```python
from build123d import *

# Parameters (mm, degrees)
BOSS_EXTRUDE1_DEPTH = 1.5
SKETCH3_W           = 30
SKETCH3_H           = 3
BOSS_EXTRUDE2_DEPTH = 3
SKETCH5_W           = 20
SKETCH5_H           = 3
BOSS_EXTRUDE3_DEPTH = 3


with BuildPart() as part:
    # Sketch2 → Boss-Extrude1 (new, symmetric)
    with BuildSketch(Plane.XY):
        with BuildLine():
            Line((-209.776110705, -9.374567854), (-209.776110705, 10.625432146))
            ThreePointArc((-209.776110705, 10.625432146), (-193.252620605, 27.63865465), (-170.374325813, 33.888382039))
            Line((-170.374325813, 33.888382039), (200.822104404, 33.888382039))
            ThreePointArc((200.822104404, 33.888382039), (223.700399196, 27.63865465), (240.223889295, 10.625432146))
            Line((240.223889295, 10.625432146), (240.223889295, -9.374567854))
            Line((240.223889295, -9.374567854), (-209.776110705, -9.374567854))
        make_face()
    extrude(amount=BOSS_EXTRUDE1_DEPTH, both=True)

    # Sketch3 → Boss-Extrude2 (add)
    with BuildSketch(Plane.XY.offset(1.5)):
        with Locations((-134.776110705, -10.874567854)):
            Rectangle(SKETCH3_W, SKETCH3_H)
        with Locations((-194.776110705, -10.874567854)):
            Rectangle(SKETCH3_W, SKETCH3_H)
        with Locations((-74.776110705, -10.874567854)):
            Rectangle(SKETCH3_W, SKETCH3_H)
        with Locations((-14.776110705, -10.874567854)):
            Rectangle(SKETCH3_W, SKETCH3_H)
        with Locations((45.223889295, -10.874567854)):
            Rectangle(SKETCH3_W, SKETCH3_H)
        with Locations((105.223889295, -10.874567854)):
            Rectangle(SKETCH3_W, SKETCH3_H)
        with Locations((165.223889295, -10.874567854)):
            Rectangle(SKETCH3_W, SKETCH3_H)
        with Locations((225.223889295, -10.874567854)):
            Rectangle(SKETCH3_W, SKETCH3_H)
    extrude(amount=-BOSS_EXTRUDE2_DEPTH)

    # Sketch5 → Boss-Extrude3 (add)
    with BuildSketch(Plane.XY.offset(1.5)):
        with Locations((-160.374325813, 35.388382039)):
            Rectangle(SKETCH5_W, SKETCH5_H)
        with Locations((-110.374325813, 35.388382039)):
            Rectangle(SKETCH5_W, SKETCH5_H)
        with Locations((-60.374325813, 35.388382039)):
            Rectangle(SKETCH5_W, SKETCH5_H)
        with Locations((-10.374325813, 35.388382039)):
            Rectangle(SKETCH5_W, SKETCH5_H)
        with Locations((39.625674187, 35.388382039)):
            Rectangle(SKETCH5_W, SKETCH5_H)
        with Locations((89.625674187, 35.388382039)):
            Rectangle(SKETCH5_W, SKETCH5_H)
        with Locations((139.625674187, 35.388382039)):
            Rectangle(SKETCH5_W, SKETCH5_H)
        with Locations((189.625674187, 35.388382039)):
            Rectangle(SKETCH5_W, SKETCH5_H)
    extrude(amount=-BOSS_EXTRUDE3_DEPTH)


solid = part.part
```
The model under review builds one solid part; all positions refer to its coordinate system, in mm. Round coordinates to 2 decimals unless told otherwise and drop trailing zeros. Order: outer loops, then holes, each group sorted by start corner. A loop starts at its lowest first (then second) coordinate and runs counter-clockwise, first axis right, second up.
(1) Wall thickness on L1, parallel to Y at x = 182, z = 0.3; L2, parallel to Y at x = 12, z = 0.2; L3, parallel to X at y = 17.5, z = 1: over which ranges is each line inside the solid? List them lowest first.
Working result:
L1: y = -9.37 to 36.89
L2: y = -9.37 to 33.89
L3: x = -205.11 to 235.56
(2) Take a section at A-A, the plane x = 7.5. State the section outline as (y, z) points.
Working result:
outline: (-9.37, -1.5) - (33.89, -1.5) - (33.89, 1.5) - (-9.37, 1.5) - close
(3) For P1, Ø1.5, axis at x = 13, z = -0.5, coming from the +Y side; P2, Ø0.9, axis at y = 36, z = 0.5, coming from the -X side; P3, Ø0.9, axis at x = -39.5, z = 0, coming from the -Y side, all flat-tipped, find the tip position at first contact; note any pin that passes through.
Working result:
P1: stops at y = 33.89
P2: stops at x = -170.37
P3: stops at y = -9.37
(4) Take a section at B-B, the plane y = 23. State the section outline as (x, z) points, plus the area to 3 significant figures.
Working result:
outline: (-199.72, -1.5) - (230.17, -1.5) - (230.17, 1.5) - (-199.72, 1.5) - close
area: 1,290 mm2
